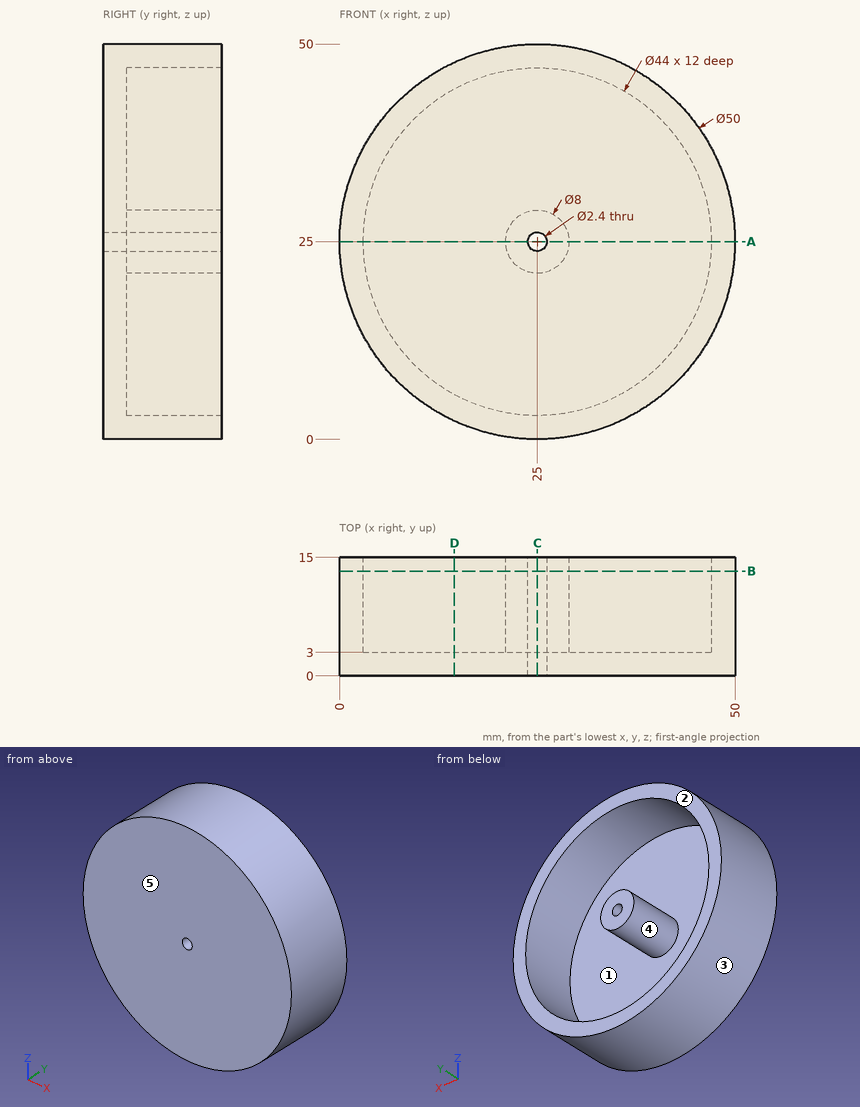
Geometry: see drawing. Coordinates: mm, zero at the bounding-box minimum. A direction names the side the tool comes from. Give positions to 0.01 mm unless a question says otherwise; leave off trailing zeros. Order: outer loops, then holes, each group sorted by start corner. A loop starts at its lowest first (then second) coordinate and runs counter-clockwise, first axis right, second up. Notation, with made-up numbers: M 10.25,-18 L 66.25,-18 A30 ccw 66.25,16 Z; hole C 21,-3 d11. An arc over 180 degrees is marked long. Answer as CSV lines item,"result". Start each with the question number.
1) Cut plane D-D (x = 14.5). Output: boundary loops of the cut face in (y, z), then the cut area to 3 significant figures.
2) Cut plane B-B (y = 13.25). Output: boundary loops of the cut face in (x, z), then the cut area to 3 significant figures.
3) Cut plane C-C (x = 25). Output: boundary loops of the cut face in (y, z), then the cut area to 3 significant figures.
4) First-contact query: P1, Ø5, axis at y = 8.5, z = 28, coming from the +X side (3 decimals); P2, Ø1.5, axis at y = 12, z = 40, coming from the +X side; P3, Ø6, axis at y = 10.5, z = 42.5, coming from the +X side. Flat tips, straight axial feed; report the tip coordinate or a pass-through.
5) Mould query, pull axis Z, two halves, no side actions, for the marked faces 3, 4 and 5. Classes: +Z half, -Z half, draft (parallel to the pull), parting line (faces both ways), or undercut.
6) Line query: line 1 (Z direction, x = 25, y = 12.25); line 2 (Z direction, x = 26, y = 11.5); line 3 (Z direction, x = 23, y = 5.5). Output: solid intervals per line, ascending. Write a range as from..to.
7) Set-up query: the marked faces 1 and 2. Return all of +Z, -Z, +X, -X, +Y, -Y with unobstructed straight access to the full face (end or side cutting, diameter ignored); none if empty.
8) Cut plane A-A (z = 25). Output: boundary loops of the cut face in (x, y).
Findings below:
1,outline,"M 0,2.31 L 15,2.31 L 15,5.67 L 3,5.67 L 3,44.33 L 15,44.33 L 15,47.69 L 0,47.69 Z"
1,area,"217 mm²"
2,outline,"C 25,25 d50; C 25,25 d8; hole C 25,25 d44; hole C 25,25 d2.4"
2,area,"489 mm²"
3,outline,"M 0,0 L 15,0 L 15,3 L 3,3 L 3,21 L 15,21 L 15,23.8 L 0,23.8 Z; M 0,26.2 L 15,26.2 L 15,29 L 3,29 L 3,47 L 15,47 L 15,50 L 0,50 Z"
3,area,"282 mm²"
4,P1,"stops at x = 49.995"
4,P2,"stops at x = 45.54"
4,P3,"stops at x = 45.37"
5,face 3,"parting line"
5,face 4,"undercut"
5,face 5,"draft"
6,line 1,"z = 0..3, 21..23.8, 26.2..29, 47..50"
6,line 2,"z = 0.02..3.02, 21.13..24.34, 25.66..28.87, 46.98..49.98"
6,line 3,"z = 0.08..3.09, 21.54..28.46, 46.91..49.92"
7,face 1,"+Y"
7,face 2,"+Z, -Z, +X, -X, +Y"
8,outline,"M 0,0 L 23.8,0 L 23.8,15 L 21,15 L 21,3 L 3,3 L 3,15 L 0,15 Z; M 26.2,0 L 50,0 L 50,15 L 47,15 L 47,3 L 29,3 L 29,15 L 26.2,15 Z"
